from build123d import *

# Parameters (mm, degrees)
F1_DEPTH = 50
F2_DEPTH = 22


with BuildPart() as f1:
    # F0 (on Front) → F1 (new body)
    with BuildSketch(Plane.XZ):
        Polygon((-15, -10), (15, -10), (15, -2), (3, 10), (-15, 10), align=None)
        Polygon((3, 10), (15, -2), (15, 10), align=None)
    extrude(amount=F1_DEPTH)

    # F0 (on Front) → F2 (cut)
    with BuildSketch(Plane.XZ):
        Polygon((3, 10), (15, -2), (15, 10), align=None)
    extrude(amount=F2_DEPTH, mode=Mode.SUBTRACT)


solid = f1.part
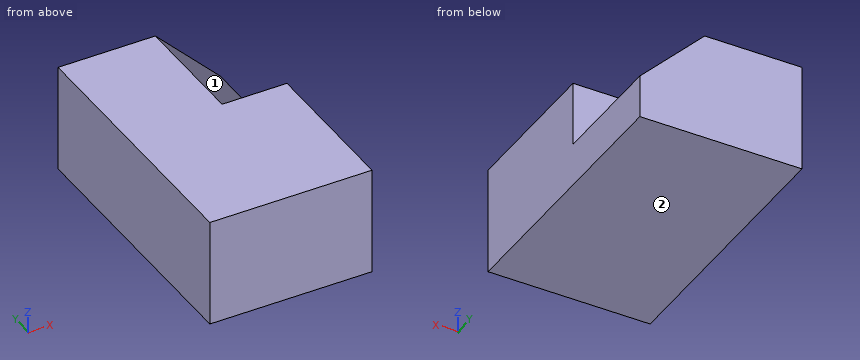
Input: part model. Units: mm. Frame: model coordinates. Face numbers are marked on the shaded views. A direction names the side the tool comes from. Coordinates: 2 decimals unless noted, no trailing zeros. Loops run counter-clockwise (first coordinate to the right, second up) from the corner with the lowest first, then second, coordinate; pieces in that order, holes last.
(1) Section C-C on x = 12.5. Return the cut outline in (y, z).
(2) Material intervals for probe 1 along Y at (x, z) = (6.75, 7.5); probe 2 along Z at (x, y) = (5, -5.5); probe 3 along X at (y, z) = (-6.5, 7.75), sorted ascending.
(3) Section B-B on y = -7.5. Return the cut outline in (x, z), then the cut area to 3 significant figures.
(4) First-contact query: pin 1 Ø8 at (y, z) = (-8, 5.5) entering from +X. Flat tip, straight axial feed; report the tip coordinate or a pass-through.
(5) Section A-A on z = 3.25. Return the cut outline in (x, y).
(6) Set-up query: the marked faces 1 and 2. Return all of +Z, -Z, +X, -X, +Y, -Y with unobstructed straight access to the full face (end or side cutting, diameter ignored); none if empty.
Data:
1. outline: (-50, -10) - (0, -10) - (0, 0.5) - (-22, 0.5) - (-22, 10) - (-50, 10) - close
2. probe 1: y = -50 to -22
2. probe 2: z = -10 to 8
2. probe 3: x = -15 to 5.25
3. outline: (-15, -10) - (15, -10) - (15, -2) - (3, 10) - (-15, 10) - close
3. area: 528 mm2
4. pin 1: stops at x = 11.5
5. outline: (-15, -50) - (15, -50) - (15, -22) - (9.75, -22) - (9.75, 0) - (-15, 0) - close
6. face 1: +Z, +X, +Y
6. face 2: -Z, +X, -X, +Y, -Y
